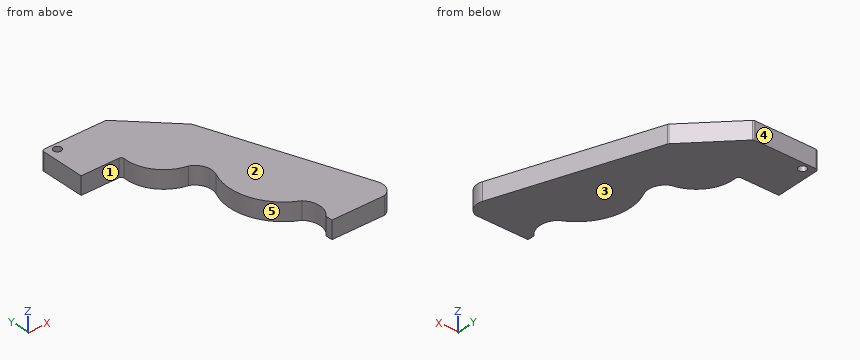
from build123d import *

# Parameters (mm, degrees)
SALIENTE_EXTRUIR1_DEPTH = 3.4
REDONDEO1_R             = 1
CROQUIS2_R              = 1.5
CORTAR_EXTRUIR1_DEPTH   = 92.234871739


with BuildPart() as part:
    # Croquis1 → Saliente-Extruir1 (new, symmetric)
    with BuildSketch(Plane.XY):
        with BuildLine():
            Line((0, 0), (0, 17.7))
            Line((0, 17.7), (24.52, 17.7))
            Line((24.52, 17.7), (42.112816716, 0.107183284))
            Line((42.112816716, 0.107183284), (63.497678713, -57.992177964))
            ThreePointArc((63.497678713, -57.992177964), (63.291104637, -62.125108825), (60.168100271, -64.84))
            Line((60.168100271, -64.84), (40.288100271, -64.84))
            Line((40.288100271, -64.84), (40.288100271, -62.22))
            ThreePointArc((40.288100271, -62.22), (42.521984385, -56.826926676), (40.288100271, -51.433853352))
            ThreePointArc((40.288100271, -51.433853352), (29.779800656, -40.049047756), (30.39958398, -24.5682846))
            ThreePointArc((30.39958398, -24.5682846), (30.487083192, -19.672969425), (27.087443921, -16.149587582))
            ThreePointArc((27.087443921, -16.149587582), (17.978818799, -10.462294263), (15.55957188, 0))
            Line((15.55957188, 0), (0, 0))
        make_face()
    extrude(amount=SALIENTE_EXTRUIR1_DEPTH, both=True)

    # Redondeo1
    redondeo1_edges = [part.edges().sort_by_distance(p)[0] for p in [
        (0, 17.7, 0),
        (24.52, 17.7, 0),
        (42.112816716, 0.107183284, 0),
        (15.55957188, 0, 0),
    ]]
    fillet(redondeo1_edges, radius=REDONDEO1_R)

    # Croquis2 → Cortar-Extruir1 (cut, through all)
    with BuildSketch(Plane.XY.offset(3.4)):
        with Locations((3.9, 15.2)):
            Circle(CROQUIS2_R)
    extrude(amount=-CORTAR_EXTRUIR1_DEPTH, mode=Mode.SUBTRACT)


solid = part.part
Read the model definition and answer for the solid it produces. Units are mm, in the model's axes. Face numbers are marked on the shaded views. A direction names the side the tool comes from. Coordinates: 2 decimals unless noted, no trailing zeros. Write each loop counter-clockwise with the first axis right and the second up, starting at its lowest first coordinate (ties: lowest second). Pieces come first, ordered by that corner, then holes. Notation, with made-up numbers: (-1, 84.5) -> (20, 84.5) arc R6 ccw to (20, 93.5) -> close; hole circle Ø11 at (84, 37.5). An arc over 180 degrees is marked (long way). Return JSON: item names as keys, results as strings.
(1) The part is cut by section D-D on y = -40. Give the vertices of the cut face in (x, z).
Answers below:
{"outline": "(29.76, -3.4) -> (56.88, -3.4) -> (56.88, 3.4) -> (29.76, 3.4) -> close"}
(2) Which of the six approach directions +Z, -Z, +X, -X, +Y, -Y give full straight-line access (tool end or side, diameter ignored) to the marked faces 1 and 2?
Answers below:
{"face 1": "+Z, -Z, -X, -Y", "face 2": "+Z, +X, -X, +Y, -Y"}
(3) The part is cut by section C-C on z = 1.5. Give the vertices of the cut face in (x, y) (1 decimal).
Answers below:
{"outline": "(0, 0) -> (14.4, 0) arc R1 cw to (15.4, -1.1) arc R14 ccw to (27.1, -16.1) arc R6.4 cw to (30.4, -24.6) arc R20.2 ccw to (40.3, -51.4) arc R7.6 cw to (40.3, -62.2) -> (40.3, -64.8) -> (60.2, -64.8) arc R5.3 ccw to (63.5, -58) -> (42.2, -0.1) arc R1 ccw to (42, 0.3) -> (24.8, 17.4) arc R1 ccw to (24.1, 17.7) -> (1, 17.7) arc R1 ccw to (0, 16.7) -> close; hole circle Ø3 at (3.9, 15.2)"}
(4) The part is cut by section A-A on x = 3.9. Give the vertices of the cut face in (y, z).
Answers below:
{"outline": "(0, -3.4) -> (13.7, -3.4) -> (13.7, 3.4) -> (0, 3.4) -> close; (16.7, -3.4) -> (17.7, -3.4) -> (17.7, 3.4) -> (16.7, 3.4) -> close"}
(5) Consider line 1 along Y through (x, z) = (3.9, -0.75); line 2 along Y through (x, z) = (37, -1.5); line 3 along X through (y, z) = (-10, -1.25). Determine where each line is inside the solid, lowest interval first. Write a range as from..to.
Answers below:
{"line 1": "0..13.7, 16.7..17.7", "line 2": "-49.52..5.22", "line 3": "17.66..45.83"}
(6) The part is cut by section B-B on y = 15.2. Give the vertices of the cut face in (x, z).
Answers below:
{"outline": "(0, -3.4) -> (2.4, -3.4) -> (2.4, 3.4) -> (0, 3.4) -> close; (5.4, -3.4) -> (27.02, -3.4) -> (27.02, 3.4) -> (5.4, 3.4) -> close"}
(7) For a pull along Y with two mould halves and no side action, classify the marked faces 3, 4 and 5 as pulls with the +Y half, pulls with the -Y half, needs draft (parallel to the pull), parting line crosses it, or undercut.
Answers below:
{"face 3": "needs draft", "face 4": "pulls with the +Y half", "face 5": "undercut"}
(8) Each of these flat-tipped pins is pushed along its axis until it touches: P1, Ø1.5, axis at y = -39, z = -0.5, coming from the +X side; P2, Ø0.8, axis at y = -63, z = -1.5, coming from the -X side; P3, Ø2, axis at x = 13.5, z = 0.5, coming from the -Y side. Where does it stop, or does it pass through?
Answers below:
{"P1": "x = 56.78", "P2": "x = 40.29", "P3": "y = 0"}
